Work out the finished part from the listing and answer in its coordinate system (mm). Face numbers are marked on the shaded views. A direction names the side the tool comes from. Give positions to 0.01 mm unless a question says otherwise; leave off trailing zeros. Order: outer loops, then holes, each group sorted by start corner. A loop starts at its lowest first (then second) coordinate and runs counter-clockwise, first axis right, second up. Notation, with made-up numbers: (66, -5) - (120, -5) arc R22 cw to (120, 33) - close; hole circle Ø8 at (26, 50). An arc over 180 degrees is marked (long way). Put each result on its own line as item: value.
Autodesk Inventor part; units mm, degrees
ref_plane "YZ Plane" through (0, 0, 0) normal (1, 0, 0) x (0, 1, 0)
ref_plane "XZ Plane" through (0, 0, 0) normal (0, 1, 0) x (-1, 0, 0)
ref_plane "XY Plane" through (0, 0, 0) normal (0, 0, 1) x (1, 0, 0)
sketch "Sketch1" plane through (0, 0, 0) normal (0, 0, 1) x (1, 0, 0)
  line L0 (-19.05, 25.4) -> (0, 25.4)
  line L1 (0, 25.4) -> (0, 0)
  line L2 (-19.05, 25.4) -> (-19.05, 22.225)
  line L3 (-19.05, 22.225) -> (-3.175, 22.225)
  line L4 (-3.175, 22.225) -> (-3.175, 3.175)
  line L5 (-3.175, 3.175) -> (-38.1, 3.175)
  line L6 (-38.1, 3.175) -> (-38.1, 0)
  line L7 (-38.1, 0) -> (0, 0)
  dimension "d2" = 3.175
  dimension "d3" = 3.175
  dimension "d4" = 3.175
  dimension "d16" = 19.05
  dimension "d17" = 38.1
  dimension "d18" = 34.925
  dimension "d19" = 15.875
  dimension "d20" = 25.4
extrude "Extrusion1" add sketch "Sketch1" against normal blind 50.8
sketch "Sketch2" plane through (-38.1, 3.175, 0) normal (0, 1, 0) x (1, 0, 0)
  line L0 (34.925, 0) -> (0, 0)
  line L1 (34.925, 0) -> (34.925, 50.8)
  circle A0 centre (12.7, 12.7) radius 4.6482
  point P0 (38.1, 0)
  dimension "d9" = 9.2964
  dimension "d10" = 22.225
  dimension "d11" = 12.7
extrude "Extrusion2" cut sketch "Sketch2" against normal blind 50.8
thread "Thread1"
sketch "Sketch3" plane through (-19.05, 25.4, 0) normal (0, 1, 0) x (1, 0, 0)
  line L0 (19.05, 50.8) -> (0, 50.8)
  line L1 (0, 0) -> (0, 50.8)
  line L2 (19.05, 0) -> (19.05, 50.8)
  line L3 (5.3975, 19.05) -> (10.4775, 19.05)
  line L4 (10.4775, 19.05) -> (10.4775, 6.35)
  line L5 (10.4775, 6.35) -> (5.3975, 6.35)
  line L6 (5.3975, 6.35) -> (5.3975, 19.05)
  arc A0 (10.4775, 19.05) -> (5.3975, 19.05) centre (7.9375, 19.05) ccw
  arc A1 (5.3975, 6.35) -> (10.4775, 6.35) centre (7.9375, 6.35) ccw
  line L7 (5.3975, 44.45) -> (10.4775, 44.45)
  line L8 (10.4775, 44.45) -> (10.4775, 31.75)
  line L9 (10.4775, 31.75) -> (5.3975, 31.75)
  line L10 (5.3975, 31.75) -> (5.3975, 44.45)
  arc A2 (10.4775, 44.45) -> (5.3975, 44.45) centre (7.9375, 44.45) ccw
  arc A3 (5.3975, 31.75) -> (10.4775, 31.75) centre (7.9375, 31.75) ccw
  dimension "d21" = 12.7
  dimension "d22" = 5.08
  dimension "d23" = 31.75
  dimension "d24" = 11.1125
  dimension "d27" = 25.4
extrude "Extrusion3" cut sketch "Sketch3" against normal blind 12.7
fillet "Fillet1" radius 6.35 4 edges at (-19.05, 23.8125, 0) (-38.1, 1.5875, 0) (-19.05, 23.8125, -50.8) (-38.1, 1.5875, -50.8)
properties part number "turn encoder mount"
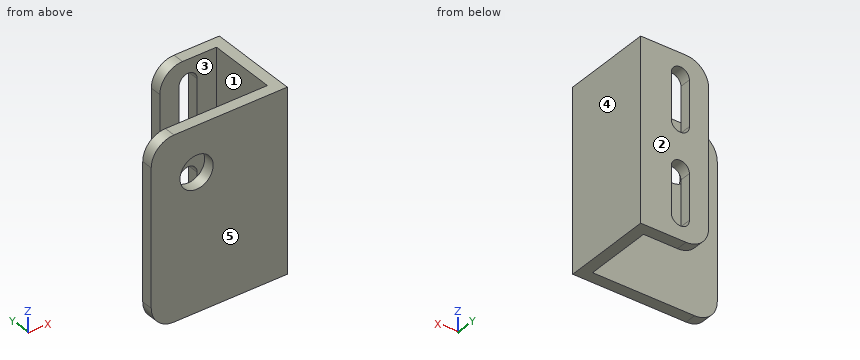
(1) Straight lines are drawn through the part: line 1 (X direction, y = 1.7, z = -12.7); line 2 (Y direction, x = -5.5, z = -4) (3 decimals); line 3 (Z direction, x = -25.4, y = 0.9). For each, find the intervals that lie inside material, in ascending order.
Geometry check:
line 1: x = -38.1 to -30.05, -20.75 to 0
line 2: y = 0 to 3.175, 22.225 to 25.4
line 3: z = -50.8 to -17.35, -8.05 to 0
(2) Section C-C, the plane y = 2.25 is taken. Write down the section's boundary in (x, z), then the cut area to 3 significant figures.
Geometry check:
outline: (-38.1, -44.45) arc R6.35 ccw to (-31.75, -50.8) - (0, -50.8) - (0, 0) - (-31.75, 0) arc R6.35 ccw to (-38.1, -6.35) - close; hole circle Ø9.3 at (-25.4, -12.7)
area: 1,850 mm²
(3) Section D-D, the plane z = -12.7 is taken. Count the separate pieces of the cut face and the enclosed holes in it, then the cut area to 3 significant figures.
Geometry check:
separate pieces: 3
enclosed holes: 0
area: 196 mm²
(4) Section A-A, the plane x = -25.4 is taken. Write down the section's boundary in (y, z) (3 decimals), then the cut area to 3 significant figures.
Geometry check:
outline: (0, -50.8) - (3.175, -50.8) - (3.175, -17.348) - (0, -17.348) - close; (0, -8.052) - (3.175, -8.052) - (3.175, 0) - (0, 0) - close
area: 132 mm²
(5) Determine the mould class of the marked faces 3, 4 and 5 for opening direction Y: pulls with the +Y half, pulls with the -Y half, needs draft (parallel to the pull), parting line crosses it, or undercut.
Geometry check:
face 3: undercut
face 4: needs draft
face 5: pulls with the -Y half
(6) Given pin 1 (2.5 mm diameter, centred on y = 23.5, z = -11, fed in from -X); pin 2 (10.5 mm diameter, centred on x = -25.4, z = -12.7, fed in from +Y) (3 decimals), each flat-ended and moving along its own axis, determine where each tip first touches the part or whether it passes through.
Geometry check:
pin 1: stops at x = -19.05
pin 2: stops at y = 3.175
(7) A tool of negligible diameter and unlimited length cuts with its end or side. For the marked faces 1 and 2, from which of +Z, -Z, +X, -X, +Y, -Y can it reach the whole face along a straight path? Write none if from no direction.
Geometry check:
face 1: +Z, -Z, -X
face 2: +Z, -Z, +X, -X, +Y
